from build123d import *

# Parameters (mm, degrees)
BOSS_EXTRUDE1_DEPTH    = 71
BOSS_EXTRUDE1_2_DEPTH  = 71
BOSS_EXTRUDE3_DEPTH    = 61
FILLET2_R              = 10
FILLET3_R              = 15
SKETCH6_R              = 25
SKETCH6_R_2            = 12.5
BOSS_EXTRUDE4_DEPTH    = 25
F_12_0MM_DOWEL_SLOT1_D = 12
F_12_0MM_DOWEL_SLOT2_D = 12


with BuildPart() as part:
    # Sketch2 → Boss-Extrude1 (new body)
    with BuildSketch(Plane.XY):
        Polygon((-43.047651623, -3.53558301), (-33.047651623, -3.53558301), (-33.047651623, -1.53558301), (-8.047651623, -1.53558301), (-8.047651623, -3.53558301), (1.952348377, -3.53558301), (1.952348377, 8.46441699), (-43.047651623, 8.46441699), align=None)
    extrude(amount=-BOSS_EXTRUDE1_DEPTH)



with BuildPart() as body_2:
    # Sketch2 → Boss-Extrude1 2 (new body)
    with BuildSketch(Plane.XY):
        Polygon((77.952348377, -3.53558301), (77.952348377, 8.46441699), (122.952348377, 8.46441699), (122.952348377, -3.53558301), (112.952348377, -3.53558301), (112.952348377, -1.53558301), (87.952348377, -1.53558301), (87.952348377, -3.53558301), align=None)
    extrude(amount=-BOSS_EXTRUDE1_2_DEPTH)


with BuildPart() as part_1:
    add(part.part)

    add(body_2.part)  # Boss-Extrude3 merges body 2
    # Sketch5 → Boss-Extrude3 (add)
    with BuildSketch(Plane.XY.offset(-10)):
        Polygon((1.952348377, 8.46441699), (1.952348377, 39.46441699), (77.952348377, 39.46441699), (77.952348377, 8.46441699), (87.952348377, 8.46441699), (87.952348377, 49.46441699), (-8.047651623, 49.46441699), (-8.047651623, 8.46441699), align=None)
    extrude(amount=-BOSS_EXTRUDE3_DEPTH)

    # Fillet2
    fillet2_edges = [part_1.edges().sort_by_distance(p)[0] for p in [
        (82.952348377, 8.46441699, -10),
        (-3.047651623, 8.46441699, -10),
    ]]
    fillet(fillet2_edges, radius=FILLET2_R - 0.0001)  # a hair under: the kernel refuses the full size

    # Fillet3
    fillet3_edges = [part_1.edges().sort_by_distance(p)[0] for p in [
        (-8.047651623, 49.46441699, -40.5),
        (87.952348377, 49.46441699, -40.5),
    ]]
    fillet(fillet3_edges, radius=FILLET3_R)

    # Sketch6 → Boss-Extrude4 (add)
    with BuildSketch(Plane(origin=(0, 49.46441699, 0), x_dir=(1, 0, 0), z_dir=(0, 1, 0))):
        with Locations(Location((39.952348377, 40, 0), (0, 0, 180))):
            Circle(SKETCH6_R)
        with Locations(Location((39.952348377, 40, 0), (0, 0, 180))):
            Circle(SKETCH6_R_2, mode=Mode.SUBTRACT)
    extrude(amount=BOSS_EXTRUDE4_DEPTH)

    # Ø12.0mm Dowel Slot1 (through all)
    with Locations(Plane(origin=(0, 8.46441699, 0), x_dir=(1, 0, 0), z_dir=(0, 1, 0))):
        with Locations((102.952348377, 48), (102.952348377, 23)):
            Hole(F_12_0MM_DOWEL_SLOT1_D / 2)

    # Ø12.0mm Dowel Slot2 (through all)
    with Locations(Plane(origin=(0, 8.46441699, 0), x_dir=(1, 0, 0), z_dir=(0, 1, 0))):
        with Locations((-23.047651623, 23), (-23.047651623, 48)):
            Hole(F_12_0MM_DOWEL_SLOT2_D / 2)


solid = part_1.part
Verification items for the finished model (mm, model axes). A direction names the side the tool comes from. Coordinates: 2 decimals unless noted, no trailing zeros. Order: outer loops, then holes, each group sorted by start corner. A loop starts at its lowest first (then second) coordinate and runs counter-clockwise, first axis right, second up.
Item 1: Access from +Z, -Z, +X, -X, +Y, -Y to the whole of each face (thin tool, end or side, straight path). Record for faces 5 (the face through (55.1, 49.464, -19.7)), 6 (the face through (39, 41, -10)), 7 (the face through (-28.59, 3.39, -20.7)), 8 (the face through (105, 8.464, -35)), 9 (the face through (-21, -1.536, -35)).
Filled in:
face 5: +Y
face 6: +Z, +X, -X, +Y
face 7: +Y, -Y
face 8: +Z, -Z, +X, +Y
face 9: +Z, -Z, -Y
Item 2: Release check for a two-part mould opening along X. For faces 1 (the face through (77.952, 18, -35)), 2 (the face through (-3, -3.536, -35)), 3 (the face through (87.952, 21, -35)), 4 (the face through (16.107, 61.789, -32.491)) record: +X half, -X half, draft (parallel to the pull), parting line (faces both ways), or undercut.
Filled in:
face 1: undercut
face 2: draft
face 3: +X half
face 4: parting line
Item 3: Depth check by flat-ended pin: pin 1 (25 mm diameter, centred on x = 35.5, y = 38.5, fed in from +Z); pin 2 (8 mm diameter, centred on y = 18.5, z = -19, fed in from -X); pin 3 (15.5 mm diameter, centred on x = -23.05, z = -48, fed in from -Y); pin 4 (12 mm diameter, centred on x = 50.5, y = 29.5, fed in from +Z). Enter the tip coordinate at first touch or a pass-through.
Filled in:
pin 1: stops at z = -10
pin 2: stops at x = -8.05
pin 3: stops at y = -1.54
pin 4: passes through
Item 4: Section check A-A, the plane y = 31. Enter the section's corners in (x, z), then the cut area to 3 significant figures.
Filled in:
outline: (-8.05, -71) - (1.95, -71) - (1.95, -10) - (-8.05, -10) - close; (77.95, -71) - (87.95, -71) - (87.95, -10) - (77.95, -10) - close
area: 1,220 mm2
Item 5: Material ranges on L1, parallel to X at y = 3, z = -23; L2, parallel to Y at x = 24, z = -51; L3, parallel to Z at x = -4.5, y = 27.5, recorded low to high.
Filled in:
L1: x = -43.05 to -29.05, -17.05 to 1.95, 77.95 to 96.95, 108.95 to 122.95
L2: y = 39.46 to 74.46
L3: z = -71 to -10
Item 6: Section check C-C, the plane z = -23. Give the number of separate pieces and of enclosed holes in the cut face, then the cut area to 3 significant figures.
Filled in:
separate pieces: 3
enclosed holes: 0
area: 3,140 mm2
Item 7: Section check D-D, the plane x = 60.5. Enter the section's corners in (y, z), then the cut area to 3 significant figures.
Filled in:
outline: (39.46, -71) - (49.46, -71) - (49.46, -54.24) - (74.46, -54.24) - (74.46, -25.76) - (49.46, -25.76) - (49.46, -10) - (39.46, -10) - close
area: 1,320 mm2
